```python
from build123d import *

# Parameters (mm, degrees)
SKETCH_1_R          = 32.5
SKETCH_1_R_2        = 11.25
EXTRUDE_1_DEPTH     = 4
EXTRUDE_START       = -4
EXTRUDE_2_DEPTH     = 4
SKETCH_3_R          = 4.15
CUT_EXTRUDE_1_DEPTH = 4
SKETCH_4_R          = 1.6
CUT_EXTRUDE_2_DEPTH = 4
SKETCH_5_W          = 17.6
SKETCH_5_H          = 4
EXTRUDE_3_DEPTH     = 4
SKETCH_6_R          = 2.1
CUT_EXTRUDE_3_DEPTH = 4
SKETCH_7_W          = 8
SKETCH_7_H          = 6
CUT_EXTRUDE_4_DEPTH = 4
FILLET_1_R          = 1
SKETCH_8_R          = 1.6
CUT_EXTRUDE_5_DEPTH = 10
SKETCH_9_W          = 35.2
SKETCH_9_H          = 4
CUT_EXTRUDE_6_DEPTH = 10
SKETCH_10_R         = 1.6
CUT_EXTRUDE_7_DEPTH = 10
EXTRUDE_4_DEPTH     = 4
FILLET_2_R          = 3
CUT_EXTRUDE_8_DEPTH = 10
EXTRUDE_5_DEPTH     = 4
FILLET_3_R          = 2
SKETCH_14_R         = 1.6
CUT_EXTRUDE_9_DEPTH = 10


with BuildPart() as part:
    # 草图1 → 凸台-拉伸1 (new body)
    with BuildSketch(Plane.XY):
        Circle(SKETCH_1_R)
        Circle(SKETCH_1_R_2, mode=Mode.SUBTRACT)
    extrude(amount=EXTRUDE_1_DEPTH)

    # 草图2 → 凸台-拉伸2 (add)
    with BuildSketch(Plane.XY.offset(4).offset(EXTRUDE_START)):
        with BuildLine():
            Line((-32.5, 0), (-32.5, -70))
            Line((-32.5, -70), (32.5, -70))
            Line((32.5, -70), (32.5, 0))
            ThreePointArc((32.5, 0), (0, -32.5), (-32.5, 0))
        make_face()
    extrude(amount=EXTRUDE_2_DEPTH)

    # 草图3 → 切除-拉伸1 (cut)
    with BuildSketch(Plane.XY.offset(4)):
        with Locations((0, 19.25)):
            Circle(SKETCH_3_R)
        with Locations((16.670989023, -9.625)):
            Circle(SKETCH_3_R)
        with Locations((-16.670989023, -9.625)):
            Circle(SKETCH_3_R)
    extrude(amount=-CUT_EXTRUDE_1_DEPTH, mode=Mode.SUBTRACT)

    # 草图4 → 切除-拉伸2 (cut)
    with BuildSketch(Plane.XY.offset(4)):
        with Locations((0, 29)):
            Circle(SKETCH_4_R)
        with Locations((25.11473671, -14.5)):
            Circle(SKETCH_4_R)
        with Locations((-25.11473671, -14.5)):
            Circle(SKETCH_4_R)
    extrude(amount=-CUT_EXTRUDE_2_DEPTH, mode=Mode.SUBTRACT)

    # 草图5 → 凸台-拉伸3 (add)
    with BuildSketch(Plane.XY.offset(4)):
        with Locations((-8.8, -72)):
            Rectangle(SKETCH_5_W, SKETCH_5_H)
        with Locations((8.8, -72)):
            Rectangle(SKETCH_5_W, SKETCH_5_H)
    extrude(amount=-EXTRUDE_3_DEPTH)

    # 草图6 → 切除-拉伸3 (cut)
    with BuildSketch(Plane.XY.offset(4)):
        with Locations((-20.5, -65)):
            Circle(SKETCH_6_R)
        with Locations((20.5, -65)):
            Circle(SKETCH_6_R)
    extrude(amount=-CUT_EXTRUDE_3_DEPTH, mode=Mode.SUBTRACT)

    # 草图7 → 切除-拉伸4 (cut)
    with BuildSketch(Plane.XY.offset(4)):
        with Locations((0, -19.2)):
            Rectangle(SKETCH_7_W, SKETCH_7_H)
    extrude(amount=-CUT_EXTRUDE_4_DEPTH, mode=Mode.SUBTRACT)

    # 圆角1
    fillet_1_edges = [part.edges().sort_by_distance(p)[0] for p in [
        (4, -16.2, 2),
        (4, -22.2, 2),
        (-4, -22.2, 2),
        (-4, -16.2, 2),
    ]]
    fillet(fillet_1_edges, radius=FILLET_1_R)

    # 草图8 → 切除-拉伸5 (cut)
    with BuildSketch(Plane(origin=(0, 0, 0), x_dir=(-1, 0, 0), z_dir=(0, 0, -1))):
        with Locations((-10, -50)):
            Circle(SKETCH_8_R)
        with Locations(Location((10, -50, 0), (0, 0, 180))):
            Circle(SKETCH_8_R)
    extrude(amount=-CUT_EXTRUDE_5_DEPTH, mode=Mode.SUBTRACT)

    # 草图9 → 切除-拉伸6 (cut)
    with BuildSketch(Plane.XY.offset(4)):
        with Locations((0, -72)):
            Rectangle(SKETCH_9_W, SKETCH_9_H)
    extrude(amount=-CUT_EXTRUDE_6_DEPTH, mode=Mode.SUBTRACT)

    # 草图10 → 切除-拉伸7 (cut)
    with BuildSketch(Plane.XY.offset(4)):
        with Locations((-29.5, -57.5)):
            Circle(SKETCH_10_R)
        with Locations((-29.5, -37.5)):
            Circle(SKETCH_10_R)
        with Locations((29.5, -37.5)):
            Circle(SKETCH_10_R)
        with Locations((29.5, -57.5)):
            Circle(SKETCH_10_R)
    extrude(amount=-CUT_EXTRUDE_7_DEPTH, mode=Mode.SUBTRACT)

    # 草图11 → 凸台-拉伸4 (add)
    with BuildSketch(Plane.XY.offset(4).offset(EXTRUDE_START)):
        with BuildLine():
            Line((12.316815341, 30.075672226), (20.846001238, 35))
            Line((20.846001238, 35), (22.961925006, 23))
            ThreePointArc((22.961925006, 23), (17.990654921, 27.06633214), (12.316815341, 30.075672226))
        make_face()
    extrude(amount=EXTRUDE_4_DEPTH)

    # 圆角2
    fillet_2_edges = [part.edges().sort_by_distance(p)[0] for p in [
        (22.961925006, 23, 2),
        (12.316815341, 30.075672226, 2),
        (20.846001238, 35, 2),
    ]]
    fillet(fillet_2_edges, radius=FILLET_2_R)

    # 草图12 → 切除-拉伸8 (cut)
    with BuildSketch(Plane.XY.offset(4)):
        with BuildLine():
            Line((-15, -27), (15, -27))
            ThreePointArc((15, -27), (17, -29), (15, -31))
            Line((15, -31), (-15, -31))
            ThreePointArc((-15, -31), (-17, -29), (-15, -27))
        make_face()
        with BuildLine():
            Line((-15, -37), (15, -37))
            ThreePointArc((15, -37), (17, -39), (15, -41))
            Line((15, -41), (-15, -41))
            ThreePointArc((-15, -41), (-17, -39), (-15, -37))
        make_face()
    extrude(amount=-CUT_EXTRUDE_8_DEPTH, mode=Mode.SUBTRACT)

    # 草图13 → 凸台-拉伸5 (add)
    with BuildSketch(Plane.XY.offset(4)):
        Polygon((-32.5, 0), (-62.5, -70), (-32.5, -70), align=None)
    extrude(amount=-EXTRUDE_5_DEPTH)

    # 圆角3
    fillet_3_edges = [part.edges().sort_by_distance(p)[0] for p in [
        (-32.5, 0, 2),
        (32.5, -70, 2),
        (-62.5, -70, 2),
    ]]
    fillet(fillet_3_edges, radius=FILLET_3_R)

    # 草图14 → 切除-拉伸9 (cut)
    with BuildSketch(Plane.XY.offset(4)):
        with Locations((-54.950382955, -60)):
            Circle(SKETCH_14_R)
        with Locations((-47.071996983, -41.6170994)):
            Circle(SKETCH_14_R)
        with Locations((-39.193611011, -23.234198799)):
            Circle(SKETCH_14_R)
        with Locations((-31.31522504, -4.851298199)):
            Circle(SKETCH_14_R)
        with BuildLine():
            Line((-33.852001481, -33.617762547), (-47.639176932, -65.787838597))
            ThreePointArc((-47.639176932, -65.787838597), (-50.265305589, -66.83829006), (-51.315757052, -64.212161403))
            Line((-51.315757052, -64.212161403), (-37.528581601, -32.042085352))
            ThreePointArc((-37.528581601, -32.042085352), (-34.902452944, -30.991633889), (-33.852001481, -33.617762547))
        make_face()
    extrude(amount=-CUT_EXTRUDE_9_DEPTH, mode=Mode.SUBTRACT)


solid = part.part
```
The model under review builds one solid part; all positions refer to its coordinate system, in mm. A direction names the side the tool comes from. Give positions to 0.01 mm unless a question says otherwise; leave off trailing zeros. Write each loop counter-clockwise with the first axis right and the second up, starting at its lowest first coordinate (ties: lowest second). Pieces come first, ordered by that corner, then holes.
(1) For P1, Ø6, axis at x = 5.5, y = -21.5, coming from the -Z side; P2, Ø2, axis at x = 3, z = 2.5, coming from the +Y side; P3, Ø1, axis at x = -41.5, z = 2.5, coming from the +Y side; P4, Ø2, axis at x = 1.5, z = 1.5, coming from the +Y side, all flat-tipped, find the tip position at first contact; note any pin that passes through.
(2) Consider section C-C, the plane y = -2. Give the boundary of the cut face in (x, z).
(3) The part is to be moulded in two halves that separate along X. For faces 3 (the cylindrical face through (-38.455, -24.654, 2.028)), 4 (the flat face through (22.187, 27.394, 1.972)), say which applies: released by +X, released by -X, zero draft, split by the parting line, or undercut.
(4) Tool access review of faces 1 (the cylindrical face through (-18.156, 26.956, 1.972)), 2 (the flat face through (-44.519, -48.352, 2.028)): name each direction out of +Z, -Z, +X, -X, +Y, -Y from which nothing blocks a thin tool from reaching the whole face with its end or side.
(5) To check wall thickness, follow L1, parallel to Y at x = 20.5, z = 2.35; L2, parallel to Y at x = 2, z = 0.8; L3, parallel to Y at x = -30, z = 1.7. State the ranges of each line that lie inside material, in increasing order.
(6) Consider section A-A, the plane x = -10. Give the boundary of the cut face in (y, z).
(7) Consider section D-D, the plane z = 0.65. Give the number of separate pieces and of enclosed holes in the cut face, and give its area (3 significant figures).
(8) Consider section B-B, the plane y = -50. Give the boundary of the cut face in (x, z).
Returned:
1. P1: stops at z = 0
1. P2: stops at y = 32.44
1. P3: stops at y = -19.83
1. P4: stops at y = 32.5
2. outline: (-33.36, 0) - (-11.07, 0) - (-11.07, 4) - (-33.36, 4) - close; (11.07, 0) - (32.5, 0) - (32.5, 4) - (11.07, 4) - close
3. face 3: undercut
3. face 4: released by +X
4. face 1: +Z, -Z, +Y
4. face 2: +Z, -Z
5. L1: y = -70 to -67.1, -62.9 to -11.23, -8.02 to 32.61
5. L2: y = -70 to -41, -37 to -31, -27 to -22.2, -16.2 to -11.07, 11.07 to 15.61, 22.89 to 32.44
5. L3: y = -70 to -59.02, -55.98 to -39.02, -35.98 to -5.76, -3.94 to 12.5
6. outline: (-70, 0) - (-51.6, 0) - (-51.6, 4) - (-70, 4) - close; (-48.4, 0) - (-41, 0) - (-41, 4) - (-48.4, 4) - close; (-37, 0) - (-31, 0) - (-31, 4) - (-37, 4) - close; (-27, 0) - (-5.15, 0) - (-5.15, 4) - (-27, 4) - close; (5.15, 0) - (30.92, 0) - (30.92, 4) - (5.15, 4) - close
7. separate pieces: 1
7. enclosed holes: 23
7. area: 6,150 mm2
8. outline: (-53.93, 0) - (-45.22, 0) - (-45.22, 4) - (-53.93, 4) - close; (-40.87, 0) - (-11.6, 0) - (-11.6, 4) - (-40.87, 4) - close; (-8.4, 0) - (8.4, 0) - (8.4, 4) - (-8.4, 4) - close; (11.6, 0) - (32.5, 0) - (32.5, 4) - (11.6, 4) - close
